from build123d import *

# Parameters (mm, degrees)
F1_DEPTH = 2
F2_R     = 1.45
F3_DEPTH = 4


with BuildPart() as f1:
    # F0 (on Top) → F1 (new body)
    with BuildSketch(Plane.XY):
        with BuildLine():
            Line((-67.440309, -11.945863), (-59.440309, -11.945863))
            ThreePointArc((-59.440309, -11.945863), (-58.733202, -11.65297), (-58.440309, -10.945863))
            Line((-58.440309, -10.945863), (-58.440309, -7.945863))
            ThreePointArc((-58.440309, -7.945863), (-58.733202, -7.238756), (-59.440309, -6.945863))
            Line((-59.440309, -6.945863), (-67.440309, -6.945863))
            ThreePointArc((-67.440309, -6.945863), (-68.147416, -7.238756), (-68.440309, -7.945863))
            Line((-68.440309, -7.945863), (-68.440309, -10.945863))
            ThreePointArc((-68.440309, -10.945863), (-68.147416, -11.65297), (-67.440309, -11.945863))
        make_face()
    extrude(amount=F1_DEPTH)

    # F2 (on face) → F3 (join)
    with BuildSketch(Plane.XY.offset(2)):
        with Locations((-60.940309, -9.445863)):
            Circle(F2_R)
    extrude(amount=F3_DEPTH)


solid = f1.part
CAD build for the part. Positions are in the model's coordinates, mm. A direction names the side the tool comes from. Give positions to 0.01 mm unless a question says otherwise; leave off trailing zeros. Order: outer loops, then holes, each group sorted by start corner. A loop starts at its lowest first (then second) coordinate and runs counter-clockwise, first axis right, second up. Notation, with made-up numbers: (41, 60) - (64, 60) arc R25 ccw to (64, 96) - close; hole circle Ø1 at (33.25, 11). An arc over 180 degrees is marked (long way). Answer in a Markdown table with one row per item.
1. Saw through at A-A, the plane z = 1.55. Give the cut face in (x, y), plus the area to 3 significant figures.
Data:
| item | result |
|---|---|
| outline | (-68.44, -10.95) arc R1 ccw to (-67.44, -11.95) - (-59.44, -11.95) arc R1 ccw to (-58.44, -10.95) - (-58.44, -7.95) arc R1 ccw to (-59.44, -6.95) - (-67.44, -6.95) arc R1 ccw to (-68.44, -7.95) - close |
| area | 49.1 mm² |
2. Saw through at C-C, the plane y = -11.05. Give the cut face in (x, z), plus the area to 3 significant figures.
Data:
| item | result |
|---|---|
| outline | (-68.43, 0) - (-58.45, 0) - (-58.45, 2) - (-68.43, 2) - close |
| area | 20.0 mm² |
3. Saw through at D-D, the plane y = -7.5. Give the cut face in (x, z), plus the area to 3 significant figures.
Data:
| item | result |
|---|---|
| outline | (-68.34, 0) - (-58.55, 0) - (-58.55, 2) - (-68.34, 2) - close |
| area | 19.6 mm² |
4. Saw through at B-B, the plane x = -62.25. Give the cut face in (y, z), plus the area to 3 significant figures.
Data:
| item | result |
|---|---|
| outline | (-11.95, 0) - (-6.95, 0) - (-6.95, 2) - (-8.82, 2) - (-8.82, 6) - (-10.07, 6) - (-10.07, 2) - (-11.95, 2) - close |
| area | 15.0 mm² |
5. Flat gauge pins, fed straight in: pin 1 (1 mm diameter, centred on x = -64.5, z = 5, fed in from -Y); pin 2 (2 mm diameter, centred on y = -8.5, z = 3.5, fed in from +X). Where does each tip first touch, or does it go through?
Data:
| item | result |
|---|---|
| pin 1 | passes through |
| pin 2 | stops at x = -59.49 |
6. Probe probe 1 along Z at (x, y) = (-62.25, -8.15); probe 2 along X at (y, z) = (-7.3, 1.25); probe 3 along X at (y, z) = (-8.15, 5.35). List the from-to ranges inside material, lowest first. Write a range as [from, to].
Data:
| item | result |
|---|---|
| probe 1 | z = [0, 2] |
| probe 2 | x = [-68.2, -58.68] |
| probe 3 | x = [-61.59, -60.29] |
7. Tool access for faces 1 (the flat face through (-68.44, -9, 1)), 2 (the cylindrical face through (-59.6, -10, 4)): list every direction of +Z, -Z, +X, -X, +Y, -Y with a clear straight run to the whole face (end or side of a thin tool).
Data:
| item | result |
|---|---|
| face 1 | +Z, -Z, -X, +Y, -Y |
| face 2 | +Z |
